```python
from build123d import *

# Parameters (mm, degrees)
SKETCH1_W                                        = 40
SKETCH1_H                                        = 40
BOSS_EXTRUDE1_DEPTH                              = 15
SKETCH2_W                                        = 30
SKETCH2_H                                        = 10
CUT_EXTRUDE1_DEPTH                               = 59.523499554
FILLET1_R                                        = 5
FILLET2_R                                        = 5
CBORE_FOR_M4_PAN_HEAD_MACHINE_SCREW1_D           = 4.3
CBORE_FOR_M4_PAN_HEAD_MACHINE_SCREW1_CBORE_D     = 8.5
CBORE_FOR_M4_PAN_HEAD_MACHINE_SCREW1_CBORE_DEPTH = 3.2
FILLET1_OF_MIRROR1_R                             = 5
FILLET2_OF_MIRROR1_R                             = 5
SKETCH4_R                                        = 3.048
CUT_EXTRUDE2_DEPTH                               = 59.523499554


with BuildPart() as part:
    # Sketch1 → Boss-Extrude1 (new body)
    with BuildSketch(Plane.XY):
        with Locations((20, 20)):
            Rectangle(SKETCH1_W, SKETCH1_H)
    boss_extrude1 = extrude(amount=BOSS_EXTRUDE1_DEPTH)

    # Sketch2 → Cut-Extrude1 (cut, through all)
    with BuildSketch(Plane.XZ):
        with Locations((15, 5)):
            Rectangle(SKETCH2_W, SKETCH2_H)
    cut_extrude1 = extrude(amount=-CUT_EXTRUDE1_DEPTH, mode=Mode.SUBTRACT)

    # Fillet1
    fillet1_edges = [part.edges().sort_by_distance(p)[0] for p in [
        (30, 20, 10),
    ]]
    fillet(fillet1_edges, radius=FILLET1_R)

    # Fillet2
    fillet2_edges = [part.edges().sort_by_distance(p)[0] for p in [
        (40, 40, 7.5),
        (40, 0, 7.5),
    ]]
    fillet(fillet2_edges, radius=FILLET2_R)

    # CBORE for M4 Pan Head Machine Screw1 (through all)
    with Locations(Plane(origin=(35, 33, 15), x_dir=(1, 0, 0), z_dir=(0, 0, 1))):
        with Locations((0, 0), (0, -26)):
            cbore_for_m4_pan_head_machine_screw1 = CounterBoreHole(CBORE_FOR_M4_PAN_HEAD_MACHINE_SCREW1_D / 2, CBORE_FOR_M4_PAN_HEAD_MACHINE_SCREW1_CBORE_D / 2, CBORE_FOR_M4_PAN_HEAD_MACHINE_SCREW1_CBORE_DEPTH)

    # Mirror1: Boss-Extrude1, Cut-Extrude1, CBORE for M4 Pan Head Machine Screw1 across plane
    add(boss_extrude1.mirror(Plane(origin=(0, 0, 15), x_dir=(0, 0, 1), z_dir=(1, 0, 0))))
    add(cut_extrude1.mirror(Plane(origin=(0, 0, 15), x_dir=(0, 0, 1), z_dir=(1, 0, 0))), mode=Mode.SUBTRACT)
    add(cbore_for_m4_pan_head_machine_screw1.mirror(Plane(origin=(0, 0, 15), x_dir=(0, 0, 1), z_dir=(1, 0, 0))), mode=Mode.SUBTRACT)

    # Fillet1 of Mirror1
    fillet1_of_mirror1_edges = [part.edges().sort_by_distance(p)[0] for p in [
        (-30, 20, 10),
    ]]
    fillet(fillet1_of_mirror1_edges, radius=FILLET1_OF_MIRROR1_R)

    # Fillet2 of Mirror1
    fillet2_of_mirror1_edges = [part.edges().sort_by_distance(p)[0] for p in [
        (-40, 40, 7.5),
        (-40, 0, 7.5),
    ]]
    fillet(fillet2_of_mirror1_edges, radius=FILLET2_OF_MIRROR1_R)

    # Sketch4 → Cut-Extrude2 (cut, through all)
    with BuildSketch(Plane.XY.offset(15)):
        with Locations((0, 20)):
            Circle(SKETCH4_R)
    extrude(amount=-CUT_EXTRUDE2_DEPTH, mode=Mode.SUBTRACT)


solid = part.part
```
Geometry check sheet. Reference: the model listing, model coordinates, mm. A direction names the side the tool comes from. Give positions to 0.01 mm unless a question says otherwise; leave off trailing zeros. Order: outer loops, then holes, each group sorted by start corner. A loop starts at its lowest first (then second) coordinate and runs counter-clockwise, first axis right, second up.
1. Access from +Z, -Z, +X, -X, +Y, -Y to the whole of each face (thin tool, end or side, straight path). Record for faces 1 (the face through (1.64, 22.57, 12.54)), 2 (the face through (28, 20, 9)), 3 (the face through (31.63, 4.41, 13.42)).
2. Thickness scan on L1, parallel to Y at x = 35, z = 14.35; L2, parallel to Y at x = -35, z = 3.5; L3, parallel to X at y = 26, z = 0.75. Record the ranges inside material, lowest first.
3. Section check B-B, the plane y = 20. Enter the section's corners in (x, z).
4. Section check A-A, the plane z = 3.5. Enter the section's corners in (x, y).
5. Section check C-C, the plane x = 0. Enter the section's corners in (y, z).
6. Gauge pin test, flat ends, axial feed: pin 1 Ø5 at (x, y) = (35, 7) entering from +Z; pin 2 Ø10 at (x, y) = (0, 20) entering from -Z. Record the tip position at first contact, or that the pin passes through.
7. Section check D-D, the plane y = 7. Enter the section's corners in (x, z), and give its area (3 significant figures).
8. Release check for a two-part mould opening along X. For faces 4 (the face through (-28, 20, 9)), 5 (the face through (-38, 1, 8)), 6 (the face through (35, 20, 0)), 7 (the face through (40, 20, 7)) record: pulls with the +X half, pulls with the -X half, needs draft (parallel to the pull), parting line crosses it, or undercut.
Values follow:
1. face 1: +Z, -Z
1. face 2: -Z, +Y, -Y
1. face 3: +Z
2. L1: y = 0 to 2.75, 11.25 to 28.75, 37.25 to 40
2. L2: y = 0 to 4.85, 9.15 to 30.85, 35.15 to 40
2. L3: x = -40 to -30, 30 to 40
3. outline: (-40, 0) - (-30, 0) - (-30, 5) arc R5 cw to (-25, 10) - (-3.05, 10) - (-3.05, 15) - (-40, 15) - close; (3.05, 10) - (25, 10) arc R5 cw to (30, 5) - (30, 0) - (40, 0) - (40, 15) - (3.05, 15) - close
4. outline: (-40, 5) arc R5 ccw to (-35, 0) - (-30, 0) - (-30, 40) - (-35, 40) arc R5 ccw to (-40, 35) - close; (30, 0) - (35, 0) arc R5 ccw to (40, 5) - (40, 35) arc R5 ccw to (35, 40) - (30, 40) - close; hole circle Ø4.3 at (-35, 7); hole circle Ø4.3 at (-35, 33); hole circle Ø4.3 at (35, 7); hole circle Ø4.3 at (35, 33)
5. outline: (0, 10) - (16.95, 10) - (16.95, 15) - (0, 15) - close; (23.05, 10) - (40, 10) - (40, 15) - (23.05, 15) - close
6. pin 1: stops at z = 11.8
6. pin 2: stops at z = 10
7. outline: (-40, 0) - (-37.15, 0) - (-37.15, 11.8) - (-39.25, 11.8) - (-39.25, 15) - (-40, 15) - close; (-32.85, 0) - (-30, 0) - (-30, 5) arc R5 cw to (-25, 10) - (25, 10) arc R5 cw to (30, 5) - (30, 0) - (32.85, 0) - (32.85, 11.8) - (30.75, 11.8) - (30.75, 15) - (-30.75, 15) - (-30.75, 11.8) - (-32.85, 11.8) - close; (37.15, 0) - (40, 0) - (40, 15) - (39.25, 15) - (39.25, 11.8) - (37.15, 11.8) - close
7. area: 455 mm2
8. face 4: undercut
8. face 5: pulls with the -X half
8. face 6: needs draft
8. face 7: pulls with the +X half
